For this review, use the dimensioned drawing (mm, ordinates from the lowest corner) and the shaded views. A direction names the side the tool comes from. Give positions to 0.01 mm unless a question says otherwise; leave off trailing zeros. Order: outer loops, then holes, each group sorted by start corner. A loop starts at its lowest first (then second) coordinate and runs counter-clockwise, first axis right, second up. Notation, with made-up numbers: M 74.25,-6.5 L 95.25,-6.5 A27 ccw 95.25,16.5 Z; hole C -37,-5 d4. An arc over 180 degrees is marked long. Use CSV: the item, a comma, the result in double quotes. Start each with the question number.
(1) Consider section D-D (x = 52). Write out the cut boundary in (y, z).
(2) Tool access review of the marked faces 1, 2 and 3: name each direction out of +Z, -Z, +X, -X, +Y, -Y from which nothing blocks a thin tool from reaching the whole face with its end or side.
(3) Clearance check with flat-ended pins moving along their axes: P1, Ø6, axis at x = 47, z = 14, coming from the +Y side; P2, Ø11, axis at y = 13, z = 35.5, coming from the +X side; P3, Ø5, axis at x = 26, z = 34, coming from the +Y side. State where each tip first meets the part, or that it passes through.
(4) Wall thickness on L1, parallel to X at y = 20.75, z = 2.5; L2, parallel to X at y = 11.25, z = 31; L3, parallel to Y at x = 57, z = 3: over which ranges is each line inside the solid? List them lowest first. Write a range as from..to.
(5) Consider section B-B (y = 19.25). Write out the cut boundary in (x, z).
(6) Consider section C-C (x = 31). Write out the cut boundary in (y, z).
(7) Consider section A-A (z = 37). Write out the cut boundary in (x, y), and give its area (3 significant figures).
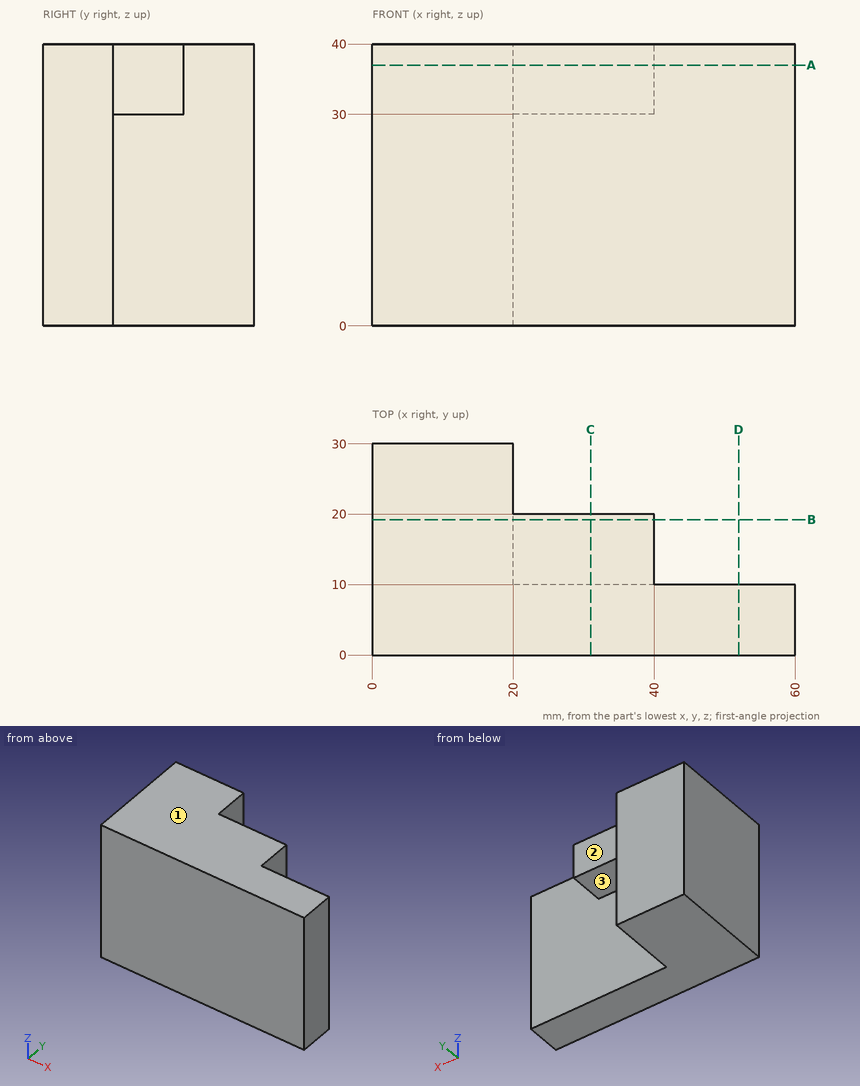
Check result:
1,outline,"M 0,0 L 10,0 L 10,40 L 0,40 Z"
2,face 1,"+Z, +X, -X, +Y, -Y"
2,face 2,"+Z, -Z, +X, +Y"
2,face 3,"-Z, +X, +Y"
3,P1,"stops at y = 10"
3,P2,"stops at x = 60"
3,P3,"stops at y = 20"
4,L1,"x = 0..20"
4,L2,"x = 0..40"
4,L3,"y = 0..10"
5,outline,"M 0,0 L 20,0 L 20,30 L 40,30 L 40,40 L 0,40 Z"
6,outline,"M 0,0 L 10,0 L 10,30 L 20,30 L 20,40 L 0,40 Z"
7,outline,"M 0,0 L 60,0 L 60,10 L 40,10 L 40,20 L 20,20 L 20,30 L 0,30 Z"
7,area,"1,200 mm^2"
